```python
from build123d import *

# Parameters (mm, degrees)
F0_W     = 45
F0_H     = 45
F1_DEPTH = 34
F2_T     = -2.4
F3_R     = 20
F4_R     = 5
F5_W     = 20
F5_H     = 24
F6_DEPTH = 5
F7_R     = 5
F9_DEPTH = 3


with BuildPart() as f1:
    # F0 (on Top) → F1 (new body)
    with BuildSketch(Plane.XY):
        Rectangle(F0_W, F0_H)
    extrude(amount=F1_DEPTH)

    # F2
    f2_openings = [f1.faces().sort_by_distance(p)[0] for p in [
        (0, 0, 34),
    ]]
    offset(amount=F2_T, openings=f2_openings)

    # F3
    f3_edges = [f1.edges().sort_by_distance(p)[0] for p in [
        (0, -20.1, 2.4),
    ]]
    fillet(f3_edges, radius=F3_R)

    # F4
    f4_edges = [f1.edges().sort_by_distance(p)[0] for p in [
        (-20.1, 10, 2.4),
        (20.1, 10, 2.4),
    ]]
    fillet(f4_edges, radius=F4_R)

    # F5 (on face) → F6 (cut)
    with BuildSketch(Plane(origin=(0, 22.5, 0), x_dir=(-1, 0, 0), z_dir=(0, 1, 0))):
        with Locations((0, 22)):
            Rectangle(F5_W, F5_H)
    extrude(amount=-F6_DEPTH, mode=Mode.SUBTRACT)

    # F7
    f7_edges = [f1.edges().sort_by_distance(p)[0] for p in [
        (10, 21.3, 10),
        (-10, 21.3, 10),
    ]]
    fillet(f7_edges, radius=F7_R)

    # F8 (on face) → F9 (cut)
    with BuildSketch(Plane(origin=(0, 0, 0), x_dir=(1, 0, 0), z_dir=(0, 0, -1))):
        Polygon((-17.5, 22.5), (-20.3, 22.5), (-20.3, 20), (-20.3, 17.5), (20.3, 17.5), (20.3, 20), (20.3, 22.5), (17.5, 22.5), (17.5, 20.3), (-17.5, 20.3), align=None)
    extrude(amount=-F9_DEPTH, mode=Mode.SUBTRACT)


solid = f1.part
```
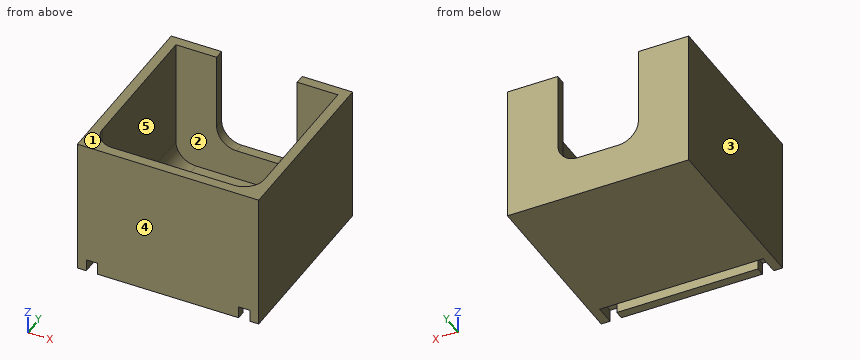
Part model, mm, in its own coordinate system. Face numbers are marked on the shaded views. A direction names the side the tool comes from. Coordinates: 2 decimals unless noted, no trailing zeros. Order: outer loops, then holes, each group sorted by start corner. A loop starts at its lowest first (then second) coordinate and runs counter-clockwise, first axis right, second up. Notation, with made-up numbers: (-6, 64.25) - (37, 64.25) arc R12 cw to (37, 71.25) - close; hole circle Ø3 at (32, 80.25). An arc over 180 degrees is marked (long way). Return JSON: item names as keys, results as strings. Group by question number.
Item 1: Pull direction X, two halves, no side cores. Call the marked faces 3, 4 and 5: pulls with the +X half, pulls with the -X half, needs draft (parallel to the pull), parting line crosses it, or undercut.
Item 2: Which spindle directions (+Z, -Z, +X, -X, +Y, -Y) get a long thin tool onto all of the face, cutting with end or side? Do the marked faces 1 and 2. Say none if no direction does.
Item 3: Drill centre lines: probe 1 along X at (y, z) = (9.5, 30.5); probe 2 along Y at (x, z) = (0, 28.5); probe 3 along Z at (x, y) = (-15, 5). Where is each one in solid material? Low to high. Write a range as from..to.
Item 4: Cut at B-B (x = -4). List the corners of the cut face in (y, z).
Item 5: Pin check, flat tips, straight feed: pin 1 (4 mm diameter, centred on x = 3.5, y = -16, fed in from +Z); pin 2 (1.5 mm diameter, centred on x = -9.5, y = -19, fed in from -Z); pin 3 (16 mm diameter, centred on x = -2, y = 12, fed in from +Z); pin 4 (1 mm diameter, centred on x = 18, y = -8.5, fed in from -Z). Stop position of each tip, or through.
Item 6: Cut at D-D (x = 16). List the corners of the cut face in (y, z).
Item 7: Cut at C-C (z = 26.5). List the corners of the cut face in (x, y), plus the area to 3 significant figures.
Item 8: Cut at A-A (y = 19). List the corners of the cut face in (x, z).
Check values:
{
 "1": {"face 3": "pulls with the -X half", "face 4": "needs draft", "face 5": "undercut"},
 "2": {"face 1": "+Z, +X, -X, +Y, -Y", "face 2": "+Z"},
 "3": {"probe 1": "x = -22.5..-20.1, 20.1..22.5", "probe 2": "y = -22.5..-20.1", "probe 3": "z = 0..2.4"},
 "4": {"outline": "(-22.5, 0) - (-20.3, 0) - (-20.3, 3) - (-17.5, 3) - (-17.5, 0) - (22.5, 0) - (22.5, 10) - (20.1, 10) - (20.1, 2.4) - (-0.1, 2.4) arc R20 cw to (-20.1, 22.4) - (-20.1, 34) - (-22.5, 34) - close"},
 "5": {"pin 1": "stops at z = 13.48", "pin 2": "stops at z = 3", "pin 3": "stops at z = 2.4", "pin 4": "stops at z = 0"},
 "6": {"outline": "(-22.5, 0) - (-20.3, 0) - (-20.3, 3) - (-17.5, 3) - (-17.5, 0) - (22.5, 0) - (22.5, 34) - (20.1, 34) - (20.1, 2.48) - (-0.1, 2.48) arc R19.92 cw to (-20.02, 22.4) - (-20.02, 34) - (-22.5, 34) - close"},
 "7": {"outline": "(-22.5, -22.5) - (22.5, -22.5) - (22.5, 22.5) - (10, 22.5) - (10, 20.1) - (20.1, 20.1) - (20.1, -15.1) arc R5 cw to (15.1, -20.1) - (-15.1, -20.1) arc R5 cw to (-20.1, -15.1) - (-20.1, 20.1) - (-10, 20.1) - (-10, 22.5) - (-22.5, 22.5) - close", "area": "372 mm2"},
 "8": {"outline": "(-22.5, 0) - (22.5, 0) - (22.5, 34) - (20.1, 34) - (20.1, 7.4) arc R5 cw to (15.1, 2.4) - (-15.1, 2.4) arc R5 cw to (-20.1, 7.4) - (-20.1, 34) - (-22.5, 34) - close"}
}
